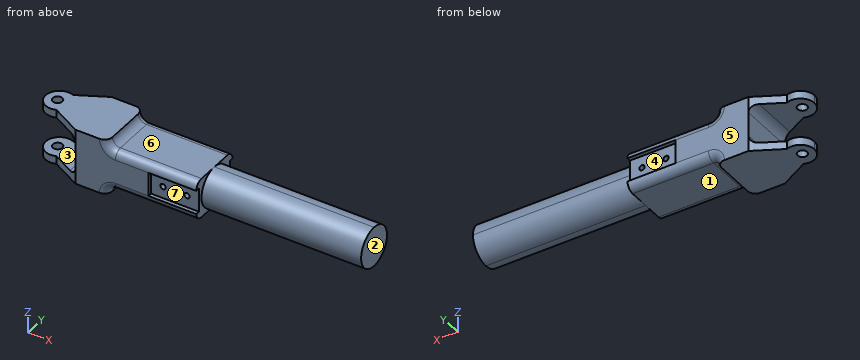
```python
from build123d import *

# Parameters (mm, degrees)
F1_DEPTH  = 35
F2_W      = 30
F2_H      = 15
F3_DEPTH  = 2.5
F4_W      = 30
F4_H      = 15
F5_DEPTH  = 2.5
F7_D      = 3.4
F8_R      = 5
F10_D     = 6
F12_DEPTH = 35
F14_DEPTH = 100


with BuildPart() as f1:
    # F0 (on Front) → F1 (new body)
    with BuildSketch(Plane.XZ):
        with BuildLine():
            Line((7.1641441025, 18.6121761102), (-12.8358558975, 18.6121761102))
            Line((-12.8358558975, 18.6121761102), (-42.8358558975, 18.6121761102))
            Line((-42.8358558975, 18.6121761102), (-42.8358558975, 13.6121761102))
            Line((-42.8358558975, 13.6121761102), (-17.8358558975, 13.6121761102))
            ThreePointArc((-17.8358558975, 13.6121761102), (-14.3003219916, 12.1477100161), (-12.8358558975, 8.6121761102))
            Line((-12.8358558975, 8.6121761102), (-12.8358558975, -6.3878238898))
            ThreePointArc((-12.8358558975, -6.3878238898), (-14.3003219916, -9.9233577957), (-17.8358558975, -11.3878238898))
            Line((-17.8358558975, -11.3878238898), (-42.8358558975, -11.3878238898))
            Line((-42.8358558975, -11.3878238898), (-42.8358558975, -16.3878238898))
            Line((-42.8358558975, -16.3878238898), (-12.8358558975, -16.3878238898))
            Line((-12.8358558975, -16.3878238898), (7.1641441025, -16.3878238898))
            ThreePointArc((7.1641441025, -16.3878238898), (8.6286101965, -12.8522899839), (12.1641441025, -11.3878238898))
            Line((12.1641441025, -11.3878238898), (62.8961617798, -11.3878238898))
            Line((62.8961617798, -11.3878238898), (62.8961617798, 13.6121761102))
            Line((62.8961617798, 13.6121761102), (12.1641441025, 13.6121761102))
            ThreePointArc((12.1641441025, 13.6121761102), (8.6286101965, 15.0766422043), (7.1641441025, 18.6121761102))
        make_face()
    extrude(amount=F1_DEPTH)

    # F2 (on face) → F3 (cut)
    with BuildSketch(Plane.XZ.offset(35)):
        with Locations((47.8961617798, 1.1121761102)):
            Rectangle(F2_W, F2_H)
    extrude(amount=-F3_DEPTH, mode=Mode.SUBTRACT)

    # F4 (on face) → F5 (cut)
    with BuildSketch(Plane(origin=(0, 0, 0), x_dir=(-1, 0, 0), z_dir=(0, 1, 0))):
        with Locations((-47.8961617798, 1.1121761102)):
            Rectangle(F4_W, F4_H)
    extrude(amount=-F5_DEPTH, mode=Mode.SUBTRACT)

    # F7 (through all)
    with Locations(Plane(origin=(0, -2.5, 0), x_dir=(-1, 0, 0), z_dir=(0, 1, 0))):
        with Locations((-55.3961617798, 1.1121761102), (-40.3961617798, 1.1121761102)):
            Hole(F7_D / 2)

    # F8
    f8_edges = [f1.edges().sort_by_distance(p)[0] for p in [
        (37.530153, 0, -11.387824),
        (37.530153, 0, 13.612176),
        (37.530153, -35, 13.612176),
        (37.530153, -35, -11.387824),
    ]]
    fillet(f8_edges, radius=F8_R)

    # F10 (through all)
    with Locations(Plane.XY.offset(18.6121761102)):
        with Locations((-35.3358558975, -17.5)):
            Hole(F10_D / 2)

    # F11 (on face) → F12 (cut)
    with BuildSketch(Plane(origin=(0, 0, -16.3878238898), x_dir=(1, 0, 0), z_dir=(0, 0, -1))):
        with BuildLine():
            Line((-42.8358558975, 0), (-12.8358558975, 0))
            Line((-12.8358558975, 0), (-30.8358558975, 9.5))
            ThreePointArc((-30.8358558975, 9.5), (-38.9765909315, 10.2888974491), (-42.8358558975, 17.5))
            Line((-42.8358558975, 17.5), (-42.8358558975, 0))
        make_face()
        with BuildLine():
            Line((-30.8358558975, 25.5), (-12.8358558975, 35))
            Line((-12.8358558975, 35), (-42.8358558975, 35))
            Line((-42.8358558975, 35), (-42.8358558975, 17.5))
            ThreePointArc((-42.8358558975, 17.5), (-38.9765909315, 24.7111025509), (-30.8358558975, 25.5))
        make_face()
    extrude(amount=-F12_DEPTH, mode=Mode.SUBTRACT)

    # F13 (on face) → F14 (join)
    with BuildSketch(Plane.YZ.offset(62.8961617798)):
        with BuildLine():
            ThreePointArc((-17.5, -11.3878238898), (-8.6611652352, -7.7266586546), (-5, 1.1121761102))
            ThreePointArc((-5, 1.1121761102), (-8.6611652352, 9.951010875), (-17.5, 13.6121761102))
            ThreePointArc((-17.5, 13.6121761102), (-30, 1.1121761102), (-17.5, -11.3878238898))
        make_face()
    extrude(amount=F14_DEPTH)


solid = f1.part
```
Geometry check sheet. Reference: the model listing, model coordinates, mm. Face numbers are marked on the shaded views. A direction names the side the tool comes from. Coordinates: 2 decimals unless noted, no trailing zeros. Loops run counter-clockwise (first coordinate to the right, second up) from the corner with the lowest first, then second, coordinate; pieces in that order, holes last.
Item 1: Sectioned sample at A-A, the plane x = 24.5. Record the boundary of the cut face in (y, z), then the cut area to 3 significant figures.
Item 2: Thickness scan on line 1 (X direction, y = -30.5, z = 0.5); line 2 (Z direction, x = -22, y = -20); line 3 (X direction, y = -4.5, z = 2.5). Record the ranges inside material, lowest first.
Item 3: Sectioned sample at B-B, the plane z = 6. Record the boundary of the cut face in (x, y).
Item 4: Sectioned sample at C-C, the plane x = 75. Record the boundary of the cut face in (y, z), then the cut area to 3 significant figures.
Item 5: Access from +Z, -Z, +X, -X, +Y, -Y to the whole of each face (thin tool, end or side, straight path). Record for the marked faces 1, 2, 3 and 4.
Item 6: Sectioned sample at D-D, the plane z = -2.5. Record the boundary of the cut face in (x, y), then the cut area to 3 significant figures.
Item 7: Go/stop test with flat-tipped pins: pin 1 Ø12 at (y, z) = (-6, -4) entering from -X; pin 2 Ø2 at (x, y) = (54.5, -34) entering from -Z; pin 3 Ø1 at (x, z) = (80, 7.5) entering from +Y; pin 4 Ø8 at (x, y) = (-35.34, -17.5) entering from -Z. Record where each tip stops, or that it passes through.
Item 8: Release check for a two-part mould opening along Z. For the marked faces 5, 6 and 7 record: released by +Z, released by -Z, zero draft, split by the parting line, or undercut.
Check result:
1. outline: (-35, -6.39) arc R5 ccw to (-30, -11.39) - (-5, -11.39) arc R5 ccw to (0, -6.39) - (0, 8.61) arc R5 ccw to (-5, 13.61) - (-30, 13.61) arc R5 ccw to (-35, 8.61) - close
1. area: 854 mm2
2. line 1: x = -12.84 to 38.81, 41.98 to 53.81, 56.98 to 62.9
2. line 2: z = -16.39 to -11.39, 13.61 to 18.61
2. line 3: x = -12.84 to 39.41, 41.38 to 54.41, 56.38 to 62.9
3. outline: (-12.84, -35) - (32.9, -35) - (32.9, -32.5) - (62.9, -32.5) - (62.9, -29) - (162.9, -29) - (162.9, -6) - (62.9, -6) - (62.9, -2.5) - (32.9, -2.5) - (32.9, 0) - (-12.84, 0) - close
4. outline: circle Ø25 at (-17.5, 1.11)
4. area: 491 mm2
5. face 1: -Z, +X, +Y, -Y
5. face 2: +Z, -Z, +X, +Y, -Y
5. face 3: -X, +Y, -Y
5. face 4: +X, +Y
6. outline: (-12.84, -35) - (32.9, -35) - (32.9, -32.5) - (62.9, -32.5) - (62.9, -29.47) - (162.9, -29.47) - (162.9, -5.53) - (62.9, -5.53) - (62.9, -2.5) - (32.9, -2.5) - (32.9, 0) - (-12.84, 0) - close
6. area: 4,890 mm2
7. pin 1: stops at x = -14.38
7. pin 2: stops at z = -10.39
7. pin 3: stops at y = -6.47
7. pin 4: stops at z = -16.39
8. face 5: zero draft
8. face 6: released by +Z
8. face 7: undercut
